CAD build for the part. Positions are in the model's coordinates, mm. Face numbers are marked on the shaded views. A direction names the side the tool comes from. Coordinates: 2 decimals unless noted, no trailing zeros. Order: outer loops, then holes, each group sorted by start corner. A loop starts at its lowest first (then second) coordinate and runs counter-clockwise, first axis right, second up. Notation, with made-up numbers: (77, -39.5) - (120, -39.5) arc R20 cw to (120, -25.5) - close; hole circle Ø9 at (74.25, 16.25). An arc over 180 degrees is marked (long way). Use one line per item in the form item = value.
```python
from build123d import *

# Parameters (mm, degrees)
SALIENTE_EXTRUIR1_DEPTH     = 100
CORTAR_EXTRUIR4_DEPTH       = 1
CORTAR_EXTRUIR4_DEPTH_BACK  = 35
CORTAR_EXTRUIR5_DEPTH       = 35
CROQUIS10_R                 = 25
CORTAR_EXTRUIR6_DEPTH       = 36
CORTAR_EXTRUIR6_DEPTH_BACK  = 66
CROQUIS12_W                 = 100
CROQUIS12_H                 = 100
CORTAR_EXTRUIR10_DEPTH      = 1
CORTAR_EXTRUIR10_DEPTH_BACK = 101
SALIENTE_EXTRUIR3_DEPTH     = 100
CROQUIS22_W                 = 100
CROQUIS22_H                 = 100
CORTAR_EXTRUIR12_DEPTH      = 35
CROQUIS23_W                 = 100
CROQUIS23_H                 = 100
CORTAR_EXTRUIR13_DEPTH      = 35
CORTAR_EXTRUIR14_DEPTH      = 36
CORTAR_EXTRUIR14_DEPTH_BACK = 66


with BuildPart() as part:
    # Croquis3 → Saliente-Extruir1 (new body)
    with BuildSketch(Plane.XY):
        with BuildLine():
            Line((-50, 100), (-50, -100))
            Line((-50, -100), (50, -100))
            Line((50, -100), (50, 100))
            ThreePointArc((50, 100), (0, 150), (-50, 100))
        make_face()
    extrude(amount=SALIENTE_EXTRUIR1_DEPTH)

    # Croquis8 → Cortar-Extruir4 (cut, two sides)
    with BuildSketch(Plane.XY.offset(100)) as cortar_extruir4_sk:
        with BuildLine():
            Line((-50, 100), (-50, 50))
            Line((-50, 50), (50, 50))
            Line((50, 50), (50, 100))
            ThreePointArc((50, 100), (0, 150), (-50, 100))
        make_face()
    extrude(amount=CORTAR_EXTRUIR4_DEPTH, mode=Mode.SUBTRACT)
    extrude(cortar_extruir4_sk.sketch, amount=-CORTAR_EXTRUIR4_DEPTH_BACK, mode=Mode.SUBTRACT)

    # Croquis9 → Cortar-Extruir5 (cut)
    with BuildSketch(Plane(origin=(0, 0, 0), x_dir=(-1, 0, 0), z_dir=(0, 0, -1))):
        with BuildLine():
            Line((-50, 100), (-50, 50))
            Line((-50, 50), (50, 50))
            Line((50, 50), (50, 100))
            ThreePointArc((50, 100), (0, 150), (-50, 100))
        make_face()
    extrude(amount=-CORTAR_EXTRUIR5_DEPTH, mode=Mode.SUBTRACT)

    # Croquis10 → Cortar-Extruir6 (cut, two sides)
    with BuildSketch(Plane(origin=(0, 0, 35), x_dir=(-1, 0, 0), z_dir=(0, 0, -1))) as cortar_extruir6_sk:
        with Locations((0, 100)):
            Circle(CROQUIS10_R)
    extrude(amount=CORTAR_EXTRUIR6_DEPTH, mode=Mode.SUBTRACT)
    extrude(cortar_extruir6_sk.sketch, amount=-CORTAR_EXTRUIR6_DEPTH_BACK, mode=Mode.SUBTRACT)

    # Croquis12 → Cortar-Extruir10 (cut, two sides)
    with BuildSketch(Plane.ZY.offset(50)) as cortar_extruir10_sk:
        with Locations((50, -50)):
            Rectangle(CROQUIS12_W, CROQUIS12_H)
    extrude(amount=CORTAR_EXTRUIR10_DEPTH, mode=Mode.SUBTRACT)
    extrude(cortar_extruir10_sk.sketch, amount=-CORTAR_EXTRUIR10_DEPTH_BACK, mode=Mode.SUBTRACT)

    # Croquis17 → Saliente-Extruir3 (add)
    with BuildSketch(Plane.ZY.offset(50)):
        with BuildLine():
            Line((0, 0), (100, 0))
            Line((100, 0), (100, -50))
            ThreePointArc((100, -50), (50, -100), (0, -50))
            Line((0, -50), (0, 0))
        make_face()
    extrude(amount=-SALIENTE_EXTRUIR3_DEPTH)

    # Croquis22 → Cortar-Extruir12 (cut)
    with BuildSketch(Plane.ZY.offset(50)):
        with Locations((50, -50)):
            Rectangle(CROQUIS22_W, CROQUIS22_H)
    extrude(amount=-CORTAR_EXTRUIR12_DEPTH, mode=Mode.SUBTRACT)

    # Croquis23 → Cortar-Extruir13 (cut)
    with BuildSketch(Plane(origin=(50, 0, 0), x_dir=(0, 0, -1), z_dir=(1, 0, 0))):
        with Locations((-50, -50)):
            Rectangle(CROQUIS23_W, CROQUIS23_H)
    extrude(amount=-CORTAR_EXTRUIR13_DEPTH, mode=Mode.SUBTRACT)

    # Croquis24 → Cortar-Extruir14 (cut, two sides)
    with BuildSketch(Plane.ZY.offset(15)) as cortar_extruir14_sk:
        with BuildLine():
            Line((25, -50), (25, -110.42880279))
            Line((25, -110.42880279), (75, -110.42880279))
            Line((75, -110.42880279), (75, -50))
            ThreePointArc((75, -50), (50, -25), (25, -50))
        make_face()
    extrude(amount=CORTAR_EXTRUIR14_DEPTH, mode=Mode.SUBTRACT)
    extrude(cortar_extruir14_sk.sketch, amount=-CORTAR_EXTRUIR14_DEPTH_BACK, mode=Mode.SUBTRACT)


solid = part.part
```
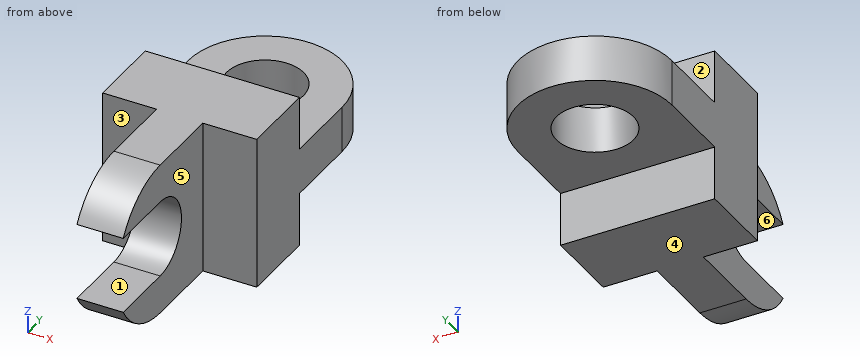
Item 1: Drop flat-ended pins along their axis: pin 1 (8 mm diameter, centred on x = 4, z = 86.5, fed in from -Y); pin 2 (5 mm diameter, centred on x = -34.5, y = 71, fed in from +Z); pin 3 (3 mm diameter, centred on y = -46.5, z = 82.5, fed in from +X). Give the stop position or say it passes through.
Derived:
pin_1 = -88
pin_2 = 65
pin_3 = 15
Item 2: 3-axis set-ups, long thin cutter, end or side, ignore diameter. For the marked faces 1, 2 and 3: which of +Z, -Z, +X, -X, +Y, -Y reach the whole face in a straight line?
Derived:
face_1 = +X, -X, -Y
face_2 = +Z, +X, -X, +Y
face_3 = +Z, -Z, -X, -Y
Item 3: Cut at A-A, the plane x = 0. Write the cut outline in (y, z), plus the area to 3 significant figures.
Derived:
outline = (-93.3, 25) arc R50 ccw to (-50, 0) - (50, 0) - (50, 35) - (75, 35) - (75, 65) - (50, 65) - (50, 100) - (-50, 100) arc R50 ccw to (-93.3, 75) - (-50, 75) arc R25 cw to (-50, 25) - close; (125, 35) - (150, 35) - (150, 65) - (125, 65) - close
area = 12,100 mm²
Item 4: Two-plate mould, pull along Z, no slides. Class the marked faces 4, 5 and 6: +Z half, -Z half, draft (parallel to the pull), parting line (faces both ways), or undercut.
Derived:
face_4 = -Z half
face_5 = draft
face_6 = undercut
Item 5: Drill centre lines: line 1 (X direction, y = -2, z = 4); line 2 (Z direction, x = 7, y = -64.5); line 3 (Z direction, x = 13.5, y = -35.5). Where is each one in solid material? Low to high. Write a range as [from, to].
Derived:
line_1 = [-15, 15]
line_2 = [2.15, 25], [75, 97.85]
line_3 = [0, 29.63], [70.37, 100]
Item 6: Cut at C-C, the plane y = 110. Write the cut outline in (x, z), plus the area to 3 significant figures.
Derived:
outline = (-48.99, 35) - (-22.91, 35) - (-22.91, 65) - (-48.99, 65) - close; (22.91, 35) - (48.99, 35) - (48.99, 65) - (22.91, 65) - close
area = 1,560 mm²
Item 7: Cut at D-D, the plane x = -22.5. Write the cut outline in (y, z), plus the area to 3 significant figures.
Derived:
outline = (0, 0) - (50, 0) - (50, 35) - (89.1, 35) - (89.1, 65) - (50, 65) - (50, 100) - (0, 100) - close; (110.9, 35) - (144.65, 35) - (144.65, 65) - (110.9, 65) - close
area = 7,190 mm²
Item 8: Cut at B-B, the plane z = 40.5. Write the cut outline in (x, y), plus the area to 3 significant figures.
Derived:
outline = (-50, 0) - (-15, 0) - (-15, -26.88) - (15, -26.88) - (15, 0) - (50, 0) - (50, 100) arc R50 ccw to (-50, 100) - close; hole circle Ø50 at (0, 100)
area = 12,800 mm²
